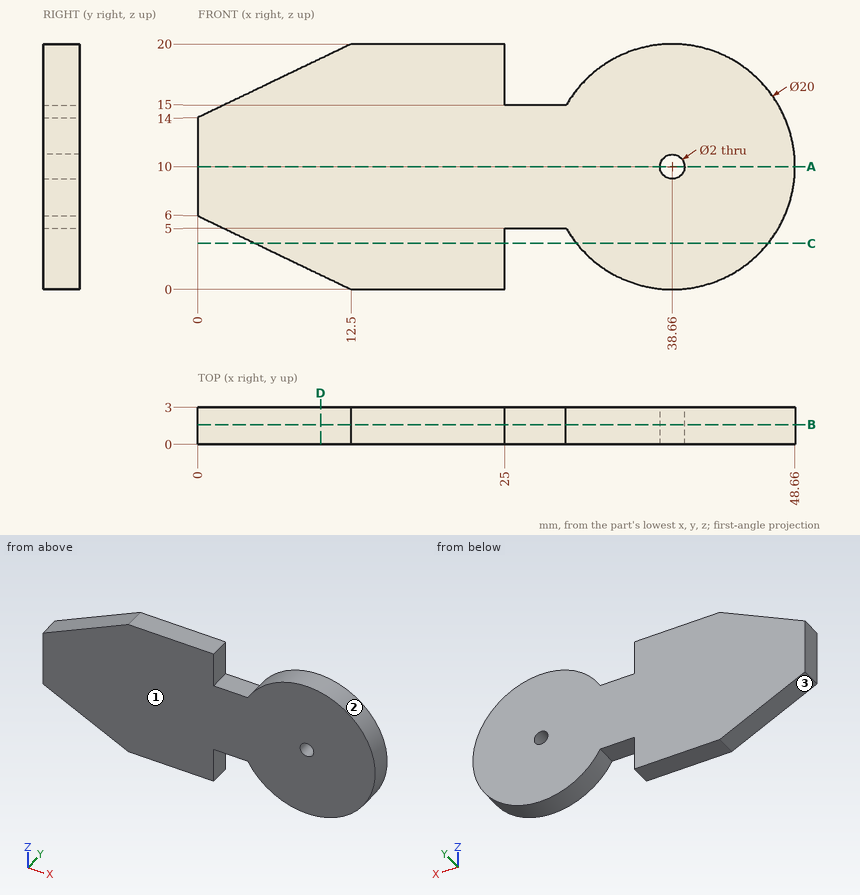
Geometry check sheet. Reference: drawing and pictorial views, mm from the part's lowest x, y, z. Coordinates: 2 decimals unless noted, no trailing zeros. Write each loop counter-clockwise with the first axis right and the second up, starting at its lowest first coordinate (ties: lowest second). Pieces come first, ordered by that corner, then holes. Notation, with made-up numbers: M 47.25,5.5 L 84.25,5.5 A17 ccw 84.25,23.5 Z; hole C 29,15.5 d7. An arc over 180 degrees is marked long. Use one line per item in the form item = value.
Item 1: Sectioned sample at C-C, the plane z = 3.75. Record the cut outline in (x, y), and give its area (3 significant figures).
Answer below:
outline = M 4.69,0 L 25,0 L 25,3 L 4.69,3 Z; M 30.85,0 L 46.47,0 L 46.47,3 L 30.85,3 Z
area = 108 mm^2
Item 2: Material ranges on L1, parallel to X at y = 1.95, z = 10; L2, parallel to Z at x = 38, y = 2.35; L3, parallel to X at y = 2.9, z = 1 (1 decimal), recorded low to high. Write a range as from..to.
Answer below:
L1 = 0..37.66, 39.66..48.66
L2 = 0.02..9.25, 10.75..19.98
L3 = 10.4..25, 34.3..43
Item 3: Gauge pin test, flat ends, axial feed: pin 1 Ø0.9 at (y, z) = (1, 2.5) entering from +X; pin 2 Ø1.5 at (x, y) = (27.5, 2) entering from +Z; pin 3 Ø10 at (x, z) = (21.5, 2) entering from -Y; pin 4 Ø0.9 at (x, y) = (28.5, 1.5) entering from -Z. Record the tip position at first contact, or that the pin passes through.
Answer below:
pin_1 = 45.75
pin_2 = 15
pin_3 = 0
pin_4 = 5
Item 4: Sectioned sample at B-B, the plane y = 1.6. Record the cut outline in (x, z).
Answer below:
outline = M 0,6 L 12.5,0 L 25,0 L 25,5 L 30,5 A10 ccw long 30,15 L 25,15 L 25,20 L 12.5,20 L 0,14 Z; hole C 38.66,10 d2
Item 5: Sectioned sample at D-D, the plane x = 10. Record the cut outline in (y, z), and give its area (3 significant figures).
Answer below:
outline = M 0,1.2 L 3,1.2 L 3,18.8 L 0,18.8 Z
area = 52.8 mm^2
Item 6: Sectioned sample at A-A, the plane z = 10. Record the cut outline in (x, y), and give its area (3 significant figures).
Answer below:
outline = M 0,0 L 37.66,0 L 37.66,3 L 0,3 Z; M 39.66,0 L 48.66,0 L 48.66,3 L 39.66,3 Z
area = 140 mm^2
Item 7: Release check for a two-part mould opening along X. For the marked faces 1, 2 and 3 record: pulls with the +X half, pulls with the -X half, needs draft (parallel to the pull), parting line crosses it, or undercut.
Answer below:
face_1 = needs draft
face_2 = undercut
face_3 = pulls with the -X half
